Source: three-view drawing plus pictorial views. Frame: mm from the lowest corner of the part. Coordinates: 2 decimals unless noted, no trailing zeros. Order: outer loops, then holes, each group sorted by start corner. A loop starts at its lowest first (then second) coordinate and runs counter-clockwise, first axis right, second up. Notation, with made-up numbers: (58.25, 43.25) - (81.25, 43.25) arc R25 ccw to (81.25, 69.25) - close; hole circle Ø1 at (-11, 72.5). An arc over 180 degrees is marked (long way). One line per question, with ' | ' between items.
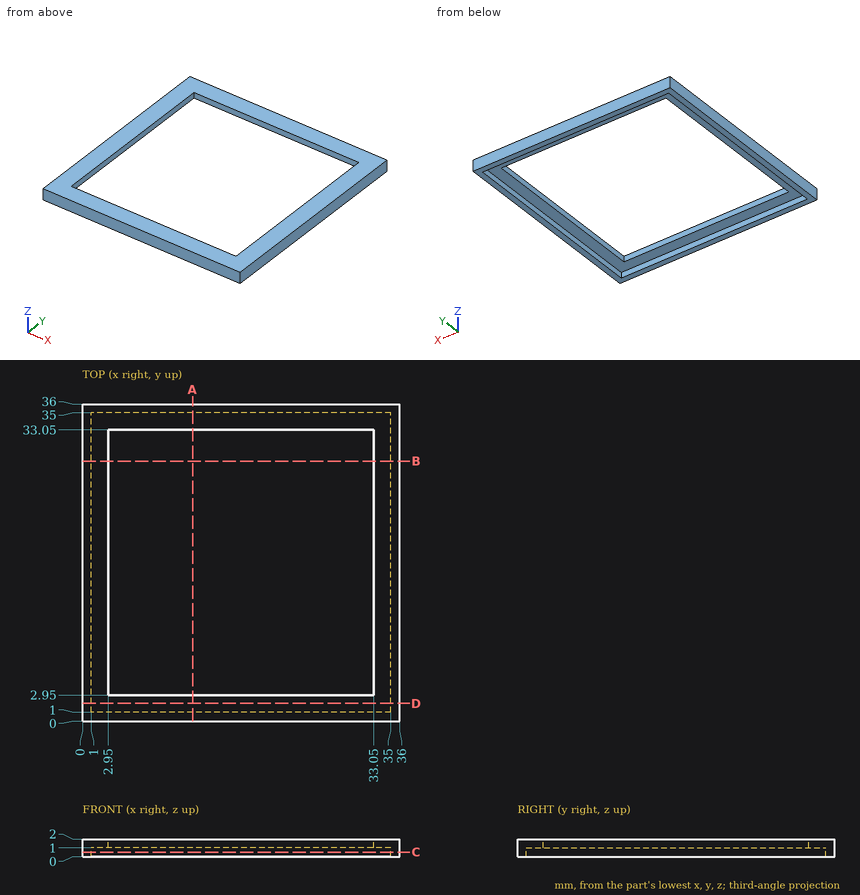
(1) Material intervals for L1, parallel to Y at x = 13, z = 1.5; L2, parallel to X at y = 22, z = 0.25, sorted ascending. Write a range as from..to.
Taken from the geometry:
L1: y = 0..2.95, 33.05..36 | L2: x = 0..1, 35..36
(2) Cut plane D-D (y = 2). Return the cut outline in (x, z).
Taken from the geometry:
outline: (0, 0) - (1, 0) - (1, 1) - (35, 1) - (35, 0) - (36, 0) - (36, 2) - (0, 2) - close
(3) Cut plane C-C (z = 0.5). Return the cut outline in (x, y), and give its area (3 significant figures).
Taken from the geometry:
outline: (0, 0) - (36, 0) - (36, 36) - (0, 36) - close; hole (1, 1) - (35, 1) - (35, 35) - (1, 35) - close | area: 140 mm²
(4) Cut plane A-A (x = 12.5). Return the cut outline in (y, z), and give its area (3 significant figures).
Taken from the geometry:
outline: (0, 0) - (1, 0) - (1, 1) - (2.95, 1) - (2.95, 2) - (0, 2) - close; (33.05, 1) - (35, 1) - (35, 0) - (36, 0) - (36, 2) - (33.05, 2) - close | area: 7.90 mm²
(5) Pin query (flat end, axial travel): P1, Ø10, axis at x = 16.5, y = 25.5, coming from the -Z side. Return the tip coordinate at first contact, or that it passes through.
Taken from the geometry:
P1: passes through
